Input: part model. Units: mm. Frame: model coordinates. A direction names the side the tool comes from. Coordinates: 2 decimals unless noted, no trailing zeros. Order: outer loops, then holes, each group sorted by start corner. A loop starts at its lowest first (then second) coordinate and runs counter-clockwise, first axis right, second up. Notation, with made-up numbers: (-10, -35.5) - (2, -35.5) arc R14 cw to (2, -24.5) - close; hole circle Ø11 at (37, -16). An arc over 180 degrees is marked (long way). One line per question, with ' | ' between items.
from build123d import *

# Parameters (mm, degrees)
BOSS_EXTRUDE1_DEPTH     = 25
CUT_EXTRUDE2_DEPTH      = 102.361975119
CUT_EXTRUDE2_DEPTH_BACK = 102.361975119
FILLET2_R               = 75
FILLET3_R               = 15
CHAMFER2_SIZE           = 2
CHAMFER3_SIZE           = 2
CHAMFER3_SIZE2          = 1.460674157
CUT_EXTRUDE3_DEPTH      = 101.57900879
CUT_EXTRUDE3_DEPTH_BACK = 101.57900879
FILLET4_R               = 2


with BuildPart() as part:
    # Sketch1 → Boss-Extrude1 (new body)
    with BuildSketch(Plane.XY):
        Polygon((0, 0), (0, 3), (45.454545455, 3), (70.909090909, 18), (95.5, 18), (95.5, 15), (75.5, 15), (75.5, -5), (45.454545455, -5), (20, -20), (20, 0), align=None)
    extrude(amount=BOSS_EXTRUDE1_DEPTH)

    # Sketch3 → Cut-Extrude2 (cut, two sides: drawn at the far end of the back side and taken through both)
    with BuildSketch(Plane(origin=(0, 3, 0), x_dir=(1, 0, 0), z_dir=(0, 1, 0)).offset(-CUT_EXTRUDE2_DEPTH_BACK)):
        with BuildLine():
            Line((6.25, -3.916666667), (13.75, -3.916666667))
            ThreePointArc((13.75, -3.916666667), (16.5, -6.666666667), (13.75, -9.416666667))
            Line((13.75, -9.416666667), (6.25, -9.416666667))
            ThreePointArc((6.25, -9.416666667), (3.5, -6.666666667), (6.25, -3.916666667))
        make_face()
        with BuildLine():
            Line((6.25, -15.583333333), (13.75, -15.583333333))
            ThreePointArc((13.75, -15.583333333), (16.5, -18.333333333), (13.75, -21.083333333))
            Line((13.75, -21.083333333), (6.25, -21.083333333))
            ThreePointArc((6.25, -21.083333333), (3.5, -18.333333333), (6.25, -15.583333333))
        make_face()
        with BuildLine():
            Line((81.75, -3.916666667), (89.25, -3.916666667))
            ThreePointArc((89.25, -3.916666667), (92, -6.666666667), (89.25, -9.416666667))
            Line((89.25, -9.416666667), (81.75, -9.416666667))
            ThreePointArc((81.75, -9.416666667), (79, -6.666666667), (81.75, -3.916666667))
        make_face()
        with BuildLine():
            Line((81.75, -15.583333333), (89.25, -15.583333333))
            ThreePointArc((89.25, -15.583333333), (92, -18.333333333), (89.25, -21.083333333))
            Line((89.25, -21.083333333), (81.75, -21.083333333))
            ThreePointArc((81.75, -21.083333333), (79, -18.333333333), (81.75, -15.583333333))
        make_face()
    extrude(amount=CUT_EXTRUDE2_DEPTH + CUT_EXTRUDE2_DEPTH_BACK, mode=Mode.SUBTRACT)

    # Fillet2
    fillet2_edges = [part.edges().sort_by_distance(p)[0] for p in [
        (45.454545455, -5, 12.5),
        (45.454545455, 3, 12.5),
    ]]
    fillet(fillet2_edges, radius=FILLET2_R)

    # Fillet3
    fillet3_edges = [part.edges().sort_by_distance(p)[0] for p in [
        (70.909090909, 18, 12.5),
    ]]
    fillet(fillet3_edges, radius=FILLET3_R)

    # Chamfer2
    chamfer2_edges = [part.edges().sort_by_distance(p)[0] for p in [
        (75.5, -5, 12.5),
    ]]
    chamfer(chamfer2_edges, length=CHAMFER2_SIZE)

    # Chamfer3
    chamfer3_edges = [part.edges().sort_by_distance(p)[0] for p in [
        (20, -20, 12.5),
    ]]
    chamfer3_side = [part.faces().sort_by_distance(p)[0] for p in [
        (20, -10, 12.5),
    ]]
    chamfer(chamfer3_edges, length=CHAMFER3_SIZE, length2=CHAMFER3_SIZE2, reference=chamfer3_side[0])

    # Sketch4 → Cut-Extrude3 (cut, two sides: drawn at the far end of the back side and taken through both)
    with BuildSketch(Plane.XY.offset(25).offset(-CUT_EXTRUDE3_DEPTH_BACK)):
        with BuildLine():
            Line((22, -2.760448796), (31.806154392, 1.301393348))
            ThreePointArc((31.806154392, 1.301393348), (28.406412173, 1.075385239), (25, 1))
            Line((25, 1), (22, 1))
            Line((22, 1), (22, -2.760448796))
        make_face()
        Polygon((42.445109464, 3.002212327), (39.283210642, -7.75), (22, -5.466429297), align=None)
        with BuildLine():
            ThreePointArc((26.816783217, -13.661538462), (30.651168911, -11.546519911), (34.599587235, -9.652896437))
            Line((34.599587235, -9.652896437), (22, -7.988156657))
            Line((22, -7.988156657), (22, -16.5))
            Line((22, -16.5), (26.816783217, -13.661538462))
        make_face()
        with BuildLine():
            ThreePointArc((42.184281307, -6.746103112), (46.856714422, -5.394323606), (51.605173683, -4.340248798))
            Line((51.605173683, -4.340248798), (45.260040246, 3.713185765))
            Line((45.260040246, 3.713185765), (42.184281307, -6.746103112))
        make_face()
        with BuildLine():
            Line((54.412012222, -3.863168035), (60.453180003, 9.647443152))
            ThreePointArc((60.453180003, 9.647443152), (54.265454394, 6.778281549), (47.848106587, 4.467938793))
            Line((47.848106587, 4.467938793), (54.412012222, -3.863168035))
        make_face()
        with BuildLine():
            Line((68.333642683, -3), (64.092307692, 11.661538462))
            Line((64.092307692, 11.661538462), (57.321727635, -3.480347675))
            ThreePointArc((57.321727635, -3.480347675), (61.608697267, -3.120180707), (65.909090909, -3))
            Line((65.909090909, -3), (68.333642683, -3))
        make_face()
        with BuildLine():
            Line((68.4, 14.2), (66.315776542, 12.971796891))
            Line((66.315776542, 12.971796891), (70.936147126, -3))
            Line((70.936147126, -3), (72.671572875, -3))
            Line((72.671572875, -3), (73.5, -2.171572875))
            Line((73.5, -2.171572875), (73.5, 15.91317157))
            ThreePointArc((73.5, 15.91317157), (70.860405913, 15.323301538), (68.4, 14.2))
        make_face()
    extrude(amount=CUT_EXTRUDE3_DEPTH + CUT_EXTRUDE3_DEPTH_BACK, mode=Mode.SUBTRACT)

    # Fillet4
    fillet4_edges = [part.edges().sort_by_distance(p)[0] for p in [
        (45.260040246, 3.713185765, 12.5),
        (54.412012222, -3.863168035, 12.5),
        (42.445109464, 3.002212327, 12.5),
        (39.283210642, -7.75, 12.5),
        (22, -5.466429297, 12.5),
        (64.092307692, 11.661538462, 12.5),
    ]]
    fillet(fillet4_edges, radius=FILLET4_R)


solid = part.part
Item 1: Section B-B on x = 23. Return the cut outline in (y, z), and give its area (3 significant figures).
Data:
outline: (-18.23, 0) - (-15.91, 0) - (-15.91, 25) - (-18.23, 25) - close; (-8.12, 0) - (-2.35, 0) - (-2.35, 25) - (-8.12, 25) - close; (1, 0) - (3, 0) - (3, 25) - (1, 25) - close | area: 252 mm^2
Item 2: Contact query for flat-ended pins moving along their axis: P1, Ø6, axis at x = 82, z = 18.5, coming from the -Y side; P2, Ø2.5, axis at x = 10, y = 1, coming from the -Z side; P3, Ø6, axis at x = 68.5, z = 11.5, coming from the -Y side; P4, Ø4, axis at y = 13, z = 15.5, coming from the -X side. Output: stop coordinate, or through.
Data:
P1: y = 15 | P2: z = 0 | P3: y = -5 | P4: x = 58.7
Item 3: Draft query along Z for faces 1 (the face through (38.95, -7.21, 12.68)), 2 (the face through (85, 16, 3.917)), 3 (the face through (48, 2, 0)). Return one class per face: released by +Z, released by -Z, zero draft, split by the parting line, or undercut.
Data:
face 1: zero draft | face 2: undercut | face 3: released by -Z
Item 4: Access query for faces 4 (the face through (10, 0, 12)), 5 (the face through (70, -5, 12)), 6 (the face through (59.624, 1.669, 12.325)), 7 (the face through (79, 16.5, 6.7)). Directions: +Z, -Z, +X, -X, +Y, -Y. A direction counts if a zero-diameter tool reaches every point of the face in a straight line with its end or side. Return the directions, or none.
Data:
face 4: +Z, -Z, -X, -Y | face 5: +Z, -Z, +X, -Y | face 6: +Z, -Z | face 7: +Y, -Y
Item 5: Section A-A on x = 70. Return the cut outline in (y, z), and give its area (3 significant figures).
Data:
outline: (-5, 0) - (0.24, 0) - (0.24, 25) - (-5, 25) - close; (15, 0) - (17.14, 0) - (17.14, 25) - (15, 25) - close | area: 184 mm^2
Item 6: Section C-C on z = 12. Count the separate pieces of the cut face and the enclosed holes in it, and give its area (3 significant figures).
Data:
separate pieces: 1 | enclosed holes: 7 | area: 661 mm^2
Item 7: Ray query, line 1 (Y direction, x = 50, z = 4); line 2 (Y direction, x = 29, z = 23.25); line 3 (Y direction, x = 28, z = 24). Return the intervals inside material, ascending.
Data:
line 1: -6.71 to -4.66, -2.3 to 1.74, 5.17 to 7.29 | line 2: -14.71 to -12.42, -8.91 to -6.35, -2.57 to 0.14, 1.1 to 3.11 | line 3: -15.29 to -12.98, -8.78 to -5.58, -3.34 to -0.28, 1.06 to 3.06
